The model under review builds one solid part; all positions refer to its coordinate system, in mm. A direction names the side the tool comes from. Round coordinates to 2 decimals unless told otherwise and drop trailing zeros. Write each loop counter-clockwise with the first axis right and the second up, starting at its lowest first coordinate (ties: lowest second). Pieces come first, ordered by that corner, then holes. Notation, with made-up numbers: (20, 20) - (39, 20) arc R27 cw to (39, 45) - close; hole circle Ø6 at (34.25, 3). An arc over 180 degrees is marked (long way). Use one line per item in the form item = value.
from build123d import *

# Parameters (mm, degrees)
F0_W         = 107.95
F0_H         = 76.2
F1_DEPTH     = 19.05
F2_W         = 3.175
F2_H         = 63.5
F3_DEPTH     = 19.051
F4_W         = 42.8625
F4_H         = 12.7
F5_DEPTH     = 9.525
F7_DEPTH     = 12.7
F8_R         = 5.08
F9_T1_DEPTH  = 2.54
F9_T6_DEPTH  = 37.7825
F9_S7_R      = 3.175
F9_T8_DEPTH  = 21
F9_T12_DEPTH = 50.4825
F9_S14_R     = 3.175
F9_T15_DEPTH = 27
F9_T17_ANGLE = 90
F9_T19_ANGLE = 90
F9_T23_DEPTH = 50.4825
F9_S25_R     = 3.175
F9_T26_DEPTH = 27
F9_T30_DEPTH = 37.7825
F9_S31_R     = 3.175
F9_T32_DEPTH = 21
F10_R        = 5.08
F11_R        = 6.35


# Not quite as in the source:
# - a fillet or chamfer that OpenCascade refuses, or shapes differently, is made with other operations: its cross-section is extruded or revolved along the edge and cut away or added


with BuildPart() as f1:
    # F0 (on Top) → F1 (new body)
    with BuildSketch(Plane.XY):
        Rectangle(F0_W, F0_H)
    extrude(amount=-F1_DEPTH)

    # F2 (on face) → F3 (cut, through all)
    with BuildSketch(Plane.XY):
        with Locations((0, 6.35)):
            Rectangle(F2_W, F2_H)
    extrude(amount=-F3_DEPTH, mode=Mode.SUBTRACT)

    # F4 (on face) → F5 (cut)
    with BuildSketch(Plane.XY):
        with Locations((23.01875, -19.05)):
            Rectangle(F4_W, F4_H)
        with Locations((-23.01875, -19.05)):
            Rectangle(F4_W, F4_H)
    extrude(amount=-F5_DEPTH, mode=Mode.SUBTRACT)

    # F6 (on face) → F7 (cut)
    with BuildSketch(Plane.XY.offset(-9.525)):
        with BuildLine():
            Line((1.5875, -15.875), (-1.5875, -15.875))
            ThreePointArc((-1.5875, -15.875), (-3.8325640303, -16.8049359697), (-4.7625, -19.05))
            ThreePointArc((-4.7625, -19.05), (-3.8325640303, -21.2950640303), (-1.5875, -22.225))
            Line((-1.5875, -22.225), (1.5875, -22.225))
            Line((1.5875, -22.225), (1.5875, -15.875))
        make_face()
        with BuildLine():
            ThreePointArc((4.7625, -19.05), (3.8325640303, -16.8049359697), (1.5875, -15.875))
            Line((1.5875, -15.875), (1.5875, -22.225))
            ThreePointArc((1.5875, -22.225), (3.8325640303, -21.2950640303), (4.7625, -19.05))
        make_face()
    extrude(amount=-F7_DEPTH, mode=Mode.SUBTRACT)

    # F8
    f8_edges = [f1.edges().sort_by_distance(p)[0] for p in [
        (-44.45, -12.7, -4.7625),
        (-44.45, -25.4, -4.7625),
        (44.45, -12.7, -4.7625),
        (44.45, -25.4, -4.7625),
    ]]
    fillet(f8_edges, radius=F8_R)

    # F9: fillet of radius 5.08 on 1 edges, made by hand

    # F9_s2 → F9_t1 (join)
    with BuildSketch(Plane.XZ.offset(17.78)):
        with BuildLine():
            ThreePointArc((44.45, -4.445), (42.9621024484, -8.0371024484), (39.37, -9.525))
            Line((39.37, -9.525), (44.45, -9.525))
            Line((44.45, -9.525), (44.45, -4.445))
        make_face()
    extrude(amount=F9_T1_DEPTH)


with BuildPart() as f9_tool4:
    # F9_s5 → F9_t6 (new body)
    with BuildSketch(Plane.YZ.offset(39.37)):
        with BuildLine():
            ThreePointArc((-12.7, -4.445), (-14.1878975516, -8.0371024484), (-17.78, -9.525))
            Line((-17.78, -9.525), (-12.7, -9.525))
            Line((-12.7, -9.525), (-12.7, -4.445))
        make_face()
    extrude(amount=-F9_T6_DEPTH)

    # F9_s7 → F9_t8 (cut, symmetric)
    with BuildSketch(Plane.XY.offset(-7)):
        with Locations((1.5875, -19.05)):
            Circle(F9_S7_R)
    extrude(amount=F9_T8_DEPTH, both=True, mode=Mode.SUBTRACT)


with BuildPart() as f1_1:
    add(f1.part)

    # F9_t3: union F9_tool4
    add(f9_tool4.part)


with BuildPart() as f9_tool10:
    # F9_s11 → F9_t12 (new body)
    with BuildSketch(Plane.YZ.offset(39.37)):
        with BuildLine():
            ThreePointArc((-12.7, -4.445), (-14.1878975516, -8.0371024484), (-17.78, -9.525))
            Line((-17.78, -9.525), (-12.7, -9.525))
            Line((-12.7, -9.525), (-12.7, -4.445))
        make_face()
    extrude(amount=-F9_T12_DEPTH)

    split(bisect_by=Plane.YZ.offset(-1.5875), keep=Keep.BOTTOM)

    # F9_s14 → F9_t15 (cut, symmetric)
    with BuildSketch(Plane.XY.offset(-7)):
        with Locations((-1.5875, -19.05)):
            Circle(F9_S14_R)
    extrude(amount=F9_T15_DEPTH, both=True, mode=Mode.SUBTRACT)


with BuildPart() as f1_2:
    add(f1_1.part)

    # F9_t9: union F9_tool10
    add(f9_tool10.part)

    # F9_s16 → F9_t17 (revolve)
    with BuildSketch(Plane.YZ.offset(39.37)):
        with BuildLine():
            ThreePointArc((-12.7, -4.445), (-14.1878975516, -8.0371024484), (-17.78, -9.525))
            Line((-17.78, -9.525), (-12.7, -9.525))
            Line((-12.7, -9.525), (-12.7, -4.445))
        make_face()
    revolve(axis=Axis((39.37, -17.78, -9.525), (0, 0, -1)), revolution_arc=F9_T17_ANGLE)

    # F9_s18 → F9_t19 (revolve)
    with BuildSketch(Plane.XZ.offset(20.32)):
        with BuildLine():
            ThreePointArc((44.45, -4.445), (42.9621024484, -8.0371024484), (39.37, -9.525))
            Line((39.37, -9.525), (44.45, -9.525))
            Line((44.45, -9.525), (44.45, -4.445))
        make_face()
    revolve(axis=Axis((39.37, -20.32, -9.525), (0, 0, -1)), revolution_arc=F9_T19_ANGLE)


with BuildPart() as f9_tool21:
    # F9_s22 → F9_t23 (new body)
    with BuildSketch(Plane.YZ.offset(-11.1125)):
        with BuildLine():
            ThreePointArc((-25.4, -4.445), (-23.9121024484, -8.0371024484), (-20.32, -9.525))
            Line((-20.32, -9.525), (-25.4, -9.525))
            Line((-25.4, -9.525), (-25.4, -4.445))
        make_face()
    extrude(amount=F9_T23_DEPTH)

    split(bisect_by=Plane.YZ.offset(-1.5875), keep=Keep.BOTTOM)

    # F9_s25 → F9_t26 (cut, symmetric)
    with BuildSketch(Plane.XY.offset(-7)):
        with Locations((-1.5875, -19.05)):
            Circle(F9_S25_R)
    extrude(amount=F9_T26_DEPTH, both=True, mode=Mode.SUBTRACT)


with BuildPart() as f1_3:
    add(f1_2.part)

    # F9_t20: union F9_tool21
    add(f9_tool21.part)


with BuildPart() as f9_tool28:
    # F9_s29 → F9_t30 (new body)
    with BuildSketch(Plane.YZ.offset(1.5875)):
        with BuildLine():
            ThreePointArc((-25.4, -4.445), (-23.9121024484, -8.0371024484), (-20.32, -9.525))
            Line((-20.32, -9.525), (-25.4, -9.525))
            Line((-25.4, -9.525), (-25.4, -4.445))
        make_face()
    extrude(amount=F9_T30_DEPTH)

    # F9_s31 → F9_t32 (cut, symmetric)
    with BuildSketch(Plane.XY.offset(-7)):
        with Locations((1.5875, -19.05)):
            Circle(F9_S31_R)
    extrude(amount=F9_T32_DEPTH, both=True, mode=Mode.SUBTRACT)


with BuildPart() as f1_4:
    add(f1_3.part)

    # F9_t27: union F9_tool28
    add(f9_tool28.part)

    # F10
    f10_edges = [f1_4.edges().sort_by_distance(p)[0] for p in [
        (-25.24125, -12.7, -9.525),
    ]]
    fillet(f10_edges, radius=F10_R)

    # F11
    f11_edges = [f1_4.edges().sort_by_distance(p)[0] for p in [
        (53.975, -38.1, -9.525),
        (53.975, 38.1, -9.525),
        (-53.975, -38.1, -9.525),
        (-53.975, 38.1, -9.525),
    ]]
    fillet(f11_edges, radius=F11_R)


solid = f1_4.part
(1) Machinability: for faces 5 (the flat face through (1.588, -24, -13)), 6 (the cylindrical face through (-6.28, -14.15, -8)), 7 (the flat face through (-13, 1, 0)), which of the approach directions +Z, -Z, +X, -X, +Y, -Y give a long, thin tool a straight path to every point of the face, cutting with its end or side? Answer none if there is none.
Geometry results:
face_5 = +Z, -Z, +Y
face_6 = +Z
face_7 = +Z, +X, -X, +Y, -Y
(2) The part is to be moulded in two halves that separate along Y. For faces 1 (the cylindrical face through (52.065, 36.289, -9.658)), 2 (the cylindrical face through (-43.001, -14.228, -2.254)), 3 (the cylindrical face through (-52.065, -36.289, -9.658)), 4 (the cylindrical face through (-42.922, -23.951, -2.254)), say which applies: +Y half, -Y half, draft (parallel to the pull), parting line (faces both ways), or undercut.
Geometry results:
face_1 = +Y half
face_2 = undercut
face_3 = -Y half
face_4 = undercut
(3) Add section C-C on x = -36. Write out the cut boundary in (y, z) (3 decimals).
Geometry results:
outline = (-38.1, -19.05) - (38.1, -19.05) - (38.1, 0) - (-12.7, 0) - (-12.7, -4.445) arc R5.08 cw to (-17.78, -9.525) - (-20.32, -9.525) arc R5.08 cw to (-25.4, -4.445) - (-25.4, 0) - (-38.1, 0) - close
(4) Insertion check: P1, Ø0.8, axis at x = 25.5, y = -19, coming from the +Z side (3 decimals); P2, Ø4, axis at x = 15.5, y = -1.5, coming from the +Z side. Each pin has a flat end and moves straight along its axis. Give the tip position at first contact, or say it passes through.
Geometry results:
P1 = -9.525
P2 = 0
(5) To check wall thickness, follow L1, parallel to X at y = 24, z = -6 (1 decimal); L2, parallel to Y at x = -38, z = -4.25; L3, parallel to Y at x = -43, z = -6. State the ranges of each line that lie inside material, in increasing order.
Geometry results:
L1 = -54 to -1.6, 1.6 to 54
L2 = -38.1 to -25.4, -12.7 to 38.1
L3 = -38.1 to -23.52, -14.58 to 38.1
